Here's how the part is built. I have some questions about the finished solid (model axes, mm). A direction names the side the tool comes from. Coordinates: 2 decimals unless noted, no trailing zeros. Loops run counter-clockwise (first coordinate to the right, second up) from the corner with the lowest first, then second, coordinate; pieces in that order, holes last. Notation, with made-up numbers: (57, 60) -> (86, 60) arc R19 cw to (86, 82) -> close; hole circle Ø3 at (2, 37). An arc over 180 degrees is marked (long way). Answer as a JSON object with one key per item and string values. Group by question number.
1) Which directions (+Z, -Z, +X, -X, +Y, -Y) give clear straight access to the entire face, cutting with the end or side of a thin tool? Please do faces 4 (the conical face through (0.19, 76.195, -0.207)), 5 (the cylindrical face through (1.438, 7.285, -0.748)), 6 (the flat face through (0, 74, -3)).
2) If we mould it in two halves opening along Z, with no side actions, what happens to faces 1 (the flat face through (0, 17, -3)), 2 (the flat face through (0, 41, 3)), 3 (the cylindrical face through (1.438, 83.715, 0.748))? For each: +Z half, -Z half, draft (parallel to the pull), parting line (faces both ways), or undercut.
3) I want a section at A-A (y = 26.5). Write out the boundary of the cut face in (x, z), then the cut area to 3 significant figures.
4) I need wall thicknesses on probe 1 along Z at (x, y) = (0, 9); probe 2 along Z at (x, y) = (3, 41); probe 3 along Y at (x, z) = (1.75, 3.5). Which ranges of each line are inside material? Lowest first, please. Write a range as [from, to].
5) I'm going to push flat-ended pins straight in: pin 1 (1.6 mm diameter, centred on x = 0.5, y = 42, fed in from +Z); pin 2 (2 mm diameter, centred on y = 31, z = 2, fed in from -X); pin 3 (2 mm diameter, centred on x = -2, y = 70, fed in from +Z). Where does each tip first touch, or does it pass through?
6) I want a section at B-B (y = 39). Write out the boundary of the cut face in (x, z), then the cut area to 3 significant figures.
Autodesk Inventor part; units mm, degrees
ref_plane "YZ Plane" through (0, 0, 0) normal (1, 0, 0) x (0, 1, 0)
ref_plane "XZ Plane" through (0, 0, 0) normal (0, 1, 0) x (-1, 0, 0)
ref_plane "XY Plane" through (0, 0, 0) normal (0, 0, 1) x (1, 0, 0)
sketch "スケッチ1" plane through (0, 0, 0) normal (0, 1, 0) x (-1, 0, 0)
  circle A0 centre (0, 0) radius 4
  dimension "d0" = 8
extrude "押し出し1" add sketch "スケッチ1" along normal blind 91
sketch "スケッチ2" plane through (0, 0, 0) normal (0, -1, 0) x (1, 0, 0)
  point P0 (0, 0)
sketch "スケッチ3" plane through (0, 91, 0) normal (0, 1, 0) x (1, 0, 0)
  point P0 (0, 0)
hole "穴1" at (0, 91, 0) direction (0, -1, 0) diameter 3.242 depth 14 tip angle 118 countersink diameter 4 countersink angle 90
hole "穴2" at (0, 0, 0) direction (0, 1, 0) diameter 3.242 depth 14 tip angle 118 countersink diameter 4 countersink angle 90
sketch "スケッチ4" plane through (0, 0, 0) normal (1, 0, 0) x (0, 1, 0)
  line L0 (76, -4) -> (76, 4)
  spline S0 degree 3 poles (39, 7.4285) (39, 7.3385) (39.0585, 7.233) (39.2835, 7.0254) (39.4498, 6.9237) (39.8139, 6.7628) (40.035, 6.6916) (40.51, 6.5961) (40.7638, 6.5723) (41.2362, 6.5723) (41.49, 6.5961) (41.965, 6.6916) (42.1861, 6.7628) (42.5502, 6.9237) (42.7165, 7.0254) (42.9415, 7.233) (43, 7.3385) (43, 7.4285) knots 0.287107 0.287107 0.287107 0.287107 0.359812 0.359812 0.432516 0.432516 0.503365 0.503365 0.574214 0.574214 0.645063 0.645063 0.715911 0.715911 0.788616 0.788616 0.861321 0.861321 0.861321 0.861321
  line L1 (15, 4) -> (15, -4)
  line L2 (76, -3) -> (72.8, -3)
  line L3 (72.8, -3) -> (72.8, -4)
  line L4 (72.8, -4) -> (76, -4)
  line L5 (44, 4) -> (38, 4)
  line L6 (38, 4) -> (38, 3)
  line L7 (38, 3) -> (44, 3)
  line L8 (44, 3) -> (44, 4)
  line L9 (43, 7.4285) -> (39, 7.4285)
  line L10 (15, -4) -> (18.2, -4)
  line L11 (18.2, -4) -> (18.2, -3)
  line L12 (18.2, -3) -> (15, -3)
  line L13 (15, -3) -> (15, -4)
  point P0 (0, 0)
  point P1 (41, 7.4285)
  point P2 (41, 4)
  dimension "d17" = 3.2
  dimension "d18" = 1
  dimension "d19" = 6
extrude "押し出し2" cut sketch "スケッチ4" along normal through all both and the other way through all contours L4 L3 L2 L0 | L12 L11 L10 L1 | L8 L7 L6 L5
properties part number "p8ALshaftP" material "アルミニウム 2014-T4"
Determined:
{
 "1": {"face 4": "+Y", "face 5": "-Y", "face 6": "-Z, +X, -X"},
 "2": {"face 1": "-Z half", "face 2": "+Z half", "face 3": "undercut"},
 "3": {"outline": "circle Ø8 at (0, 0)", "area": "50.3 mm^2"},
 "4": {"probe 1": "[-4, -1.62], [1.62, 4]", "probe 2": "[-2.65, 2.65]", "probe 3": "[0, 38], [44, 91]"},
 "5": {"pin 1": "z = 3", "pin 2": "x = -3.87", "pin 3": "z = 3.87"},
 "6": {"outline": "(-2.65, 3) arc R4 ccw (long way) to (2.65, 3) -> close", "area": "46.6 mm^2"}
}
